The listing builds one solid part. Answer for the finished solid, in the listing's coordinates (mm). A direction names the side the tool comes from. Give positions to 0.01 mm unless a question says otherwise; leave off trailing zeros. Write each loop counter-clockwise with the first axis right and the second up, starting at its lowest first coordinate (ties: lowest second). Pieces come first, ordered by that corner, then holes. Notation, with made-up numbers: (-32, -7) - (-14, -7) arc R8 cw to (-14, 7) - close; hole circle Ø2 at (-32, -37). An arc over 180 degrees is marked (long way). Write each question's results on one line, items separated by ' | '. Start each with the question number.
Q1. Find the intervals of material crossed by probe 1 along Y at (x, z) = (64.21, 0.2); probe 2 along X at (y, z) = (29.5, 7.75); probe 3 along Y at (x, z) = (18.5, 5), in increasing order.
Q2. Section C-C (z = 6) is taken. Determine the outline of the cut face in (x, y).
Q3. Section A-A (y = -3) is taken. Determine the outline of the cut face in (x, z), plus the area to 3 significant figures.
Q4. For a pull along X with two mould halves and no side action, classify faces 3 (the face through (-63.28, -30.7, 0.25)), 4 (the face through (97.044, -55.784, 5.423)), 5 (the face through (-96.684, -55.644, 5.423)) as pulls with the +X half, pulls with the -X half, needs draft (parallel to the pull), parting line crosses it, or undercut.
Q5. Flat-ended cylindrical pins translate along their axes: pin 1 Ø3.5 at (x, y) = (64, -33.5) entering from +Z; pin 2 Ø10 at (x, y) = (57.5, 41.5) entering from +Z; pin 3 Ø2 at (x, y) = (-61.99, 33.77) entering from +Z. Find the tip coordinate at first contact, or state that the pin passes through.
Q6. Section B-B (x = -49.5) is taken. Determine the outline of the cut face in (y, z), plus the area to 3 significant figures.
Q7. For faces 1 (the face through (-1, 48, 3)), 2 (the face through (-99.25, 1, 5)), determine the directions among +Z, -Z, +X, -X, +Y, -Y from which every point of the face is accessible in a straight line to the end or side of a thin tool.
```python
from build123d import *

# Parameters (mm, degrees)
F1_DEPTH  = 12
F2_R      = 1.75
F3_DEPTH  = 25
F4_R      = 1.75
F5_DEPTH  = 3
F6_R      = 1
F7_W      = 167.5
F7_H      = 105.3
F8_DEPTH  = 6
F9_W      = 107.5
F9_H      = 92.3
F10_DEPTH = 6
F11_R     = 6
F12_DEPTH = 2.5


with BuildPart() as f1:
    # F0 (on Top) → F1 (new body)
    with BuildSketch(Plane.XY):
        with BuildLine():
            Line((90.75, 58.35), (-90.25, 58.35))
            ThreePointArc((-90.25, 58.35), (-96.613961, 55.713961), (-99.25, 49.35))
            Line((-99.25, 49.35), (-99.25, -49.35))
            ThreePointArc((-99.25, -49.35), (-96.613961, -55.713961), (-90.25, -58.35))
            Line((-90.25, -58.35), (90.75, -58.35))
            ThreePointArc((90.75, -58.35), (97.113961, -55.713961), (99.75, -49.35))
            Line((99.75, -49.35), (99.75, 49.35))
            ThreePointArc((99.75, 49.35), (97.113961, 55.713961), (90.75, 58.35))
        make_face()
    extrude(amount=F1_DEPTH)

    # F2 (on face) → F3 (cut)
    with BuildSketch(Plane.XY.offset(12)):
        with Locations((-61.99, 33.77)):
            Circle(F2_R)
        with Locations((64.21, 33.77)):
            Circle(F2_R)
        with Locations((64.21, -31.88)):
            Circle(F2_R)
        with Locations((-61.99, -31.88)):
            Circle(F2_R)
    extrude(amount=-F3_DEPTH, mode=Mode.SUBTRACT)

    # F4 (on face) → F5 (cut)
    with BuildSketch(Plane.XY.offset(12)):
        with BuildLine():
            Line((90.75, 55.95), (-90.75, 55.95))
            ThreePointArc((-90.75, 55.95), (-94.992641, 54.192641), (-96.75, 49.95))
            Line((-96.75, 49.95), (-96.75, -49.35))
            ThreePointArc((-96.75, -49.35), (-94.992641, -53.592641), (-90.75, -55.35))
            Line((-90.75, -55.35), (90.75, -55.35))
            ThreePointArc((90.75, -55.35), (94.992641, -53.592641), (96.75, -49.35))
            Line((96.75, -49.35), (96.75, 49.95))
            ThreePointArc((96.75, 49.95), (94.992641, 54.192641), (90.75, 55.95))
        make_face()
        with Locations((-61.99, -31.88)):
            Circle(F4_R, mode=Mode.SUBTRACT)
        with Locations((64.21, -31.88)):
            Circle(F4_R, mode=Mode.SUBTRACT)
        with Locations((-61.99, 33.77)):
            Circle(F4_R, mode=Mode.SUBTRACT)
        with Locations((64.21, 33.77)):
            Circle(F4_R, mode=Mode.SUBTRACT)
    extrude(amount=-F5_DEPTH, mode=Mode.SUBTRACT)

    # F6
    f6_edges = [f1.edges().sort_by_distance(p)[0] for p in [
        (-99.25, 0, 12),
        (-96.75, 0.3, 12),
        (-96.613961, 55.713961, 12),
        (0, 55.95, 12),
        (0.25, 58.35, 12),
        (94.992641, 54.192641, 12),
        (99.75, 0, 12),
        (96.75, 0.3, 12),
        (97.113961, -55.713961, 12),
        (94.992641, -53.592641, 12),
        (0.25, -58.35, 12),
        (0, -55.35, 12),
        (-94.992641, -53.592641, 12),
        (-96.613961, -55.713961, 12),
        (97.113961, 55.713961, 12),
        (-94.992641, 54.192641, 12),
    ]]
    fillet(f6_edges, radius=F6_R)

    # F7 (on face) → F8 (cut)
    with BuildSketch(Plane.XY.offset(9)):
        with Locations((0, 0.3)):
            Rectangle(F7_W, F7_H)
    extrude(amount=-F8_DEPTH, mode=Mode.SUBTRACT)

    # F9 (on face) → F10 (cut)
    with BuildSketch(Plane.XY.offset(3)):
        with Locations((0, -6.2)):
            Rectangle(F9_W, F9_H)
    extrude(amount=-F10_DEPTH, mode=Mode.SUBTRACT)

    # F11 (on face) → F12 (cut)
    with BuildSketch(Plane.XY.offset(3)):
        with Locations((-61.99, 33.77)):
            Circle(F11_R)
        with Locations((-61.99, -31.88)):
            Circle(F11_R)
        with Locations((64.21, 33.77)):
            Circle(F11_R)
        with Locations((64.21, -31.88)):
            Circle(F11_R)
    extrude(amount=-F12_DEPTH, mode=Mode.SUBTRACT)


solid = f1.part
```
Answers below:
1) probe 1: y = -58.35 to -33.63, -30.13 to 32.02, 35.52 to 58.35 | probe 2: x = -99.25 to -83.75, 83.75 to 99.75 | probe 3: y = -58.35 to -52.35, 52.95 to 58.35
2) outline: (-99.25, -49.35) arc R9 ccw to (-90.25, -58.35) - (90.75, -58.35) arc R9 ccw to (99.75, -49.35) - (99.75, 49.35) arc R9 ccw to (90.75, 58.35) - (-90.25, 58.35) arc R9 ccw to (-99.25, 49.35) - close; hole (-83.75, -52.35) - (83.75, -52.35) - (83.75, 52.95) - (-83.75, 52.95) - close
3) outline: (-99.25, 0) - (-53.75, 0) - (-53.75, 3) - (-83.75, 3) - (-83.75, 9) - (-96.75, 9) - (-96.75, 11) arc R1 ccw to (-97.75, 12) - (-98.25, 12) arc R1 ccw to (-99.25, 11) - close; (53.75, 0) - (99.75, 0) - (99.75, 11) arc R1 ccw to (98.75, 12) - (97.75, 12) arc R1 ccw to (96.75, 11) - (96.75, 9) - (83.75, 9) - (83.75, 3) - (53.75, 3) - close | area: 479 mm2
4) face 3: undercut | face 4: pulls with the +X half | face 5: pulls with the -X half
5) pin 1: stops at z = 0.5 | pin 2: stops at z = 3 | pin 3: passes through
6) outline: (-58.35, 0) - (-52.35, 0) - (-52.35, 9) - (-55.35, 9) - (-55.35, 11) arc R1 ccw to (-56.35, 12) - (-57.35, 12) arc R1 ccw to (-58.35, 11) - close; (39.95, 0) - (58.35, 0) - (58.35, 11) arc R1 ccw to (57.35, 12) - (56.95, 12) arc R1 ccw to (55.95, 11) - (55.95, 9) - (52.95, 9) - (52.95, 3) - (39.95, 3) - close | area: 157 mm2
7) face 1: +Z | face 2: +Z, -Z, -X, +Y, -Y
